Geometry: final body of the model. Coordinates: model frame, mm. A direction names the side the tool comes from. Give positions to 0.01 mm unless a question says otherwise; leave off trailing zeros. Loops run counter-clockwise (first coordinate to the right, second up) from the corner with the lowest first, then second, coordinate; pieces in that order, holes last. Notation, with made-up numbers: (4, -38) -> (29, -38) arc R18 ccw to (29, -7) -> close; hole circle Ø7 at (-30.5, 24.25). An arc over 180 degrees is marked (long way). One line per item, written item: value. Start each with the question number.
from build123d import *
from build123d.topology import SkipClean

# Parameters (mm, degrees)
SALIENTE_EXTRUIR1_DEPTH    = 2.4
CORTAR_EXTRUIR1_DEPTH      = 43.673293756
CORTAR_EXTRUIR1_DEPTH_BACK = 43.673293756
CROQUIS2_R                 = 1.5
CROQUIS3_R                 = 1.5
SALIENTE_EXTRUIR2_DEPTH    = 7.5
CORTAR_EXTRUIR2_DEPTH      = 3.1
REDONDEO1_R                = 2


with BuildPart() as part:
    # Croquis1 → Saliente-Extruir1 (new, symmetric)
    with BuildSketch(Plane(origin=(0, 0, 0), x_dir=(0, 0, -1), z_dir=(1, 0, 0))):
        with BuildLine():
            Line((-41.5, 3), (41.5, 3))
            ThreePointArc((41.5, 3), (42.207106781, 2.707106781), (42.5, 2))
            Line((42.5, 2), (42.5, -2))
            ThreePointArc((42.5, -2), (42.207106781, -2.707106781), (41.5, -3))
            Line((41.5, -3), (-41.5, -3))
            ThreePointArc((-41.5, -3), (-42.207106781, -2.707106781), (-42.5, -2))
            Line((-42.5, -2), (-42.5, 2))
            ThreePointArc((-42.5, 2), (-42.207106781, 2.707106781), (-41.5, 3))
        make_face()
    extrude(amount=SALIENTE_EXTRUIR1_DEPTH, both=True)

    # Croquis2 → Cortar-Extruir1 (cut, two sides: drawn at the far end of the back side and taken through both)
    with BuildSketch(Plane(origin=(0, 0, 0), x_dir=(0, 0, -1), z_dir=(1, 0, 0)).offset(-CORTAR_EXTRUIR1_DEPTH_BACK)):
        with Locations((-39.5, 0)):
            Circle(CROQUIS2_R)
        with Locations((33.5, 0)):
            Circle(CROQUIS2_R)
    extrude(amount=CORTAR_EXTRUIR1_DEPTH + CORTAR_EXTRUIR1_DEPTH_BACK, mode=Mode.SUBTRACT)

    # Croquis3 → Saliente-Extruir2 (add, symmetric)
    with SkipClean():  # the faces are left unmerged after this step: merging them gives an invalid solid
        with BuildSketch(Plane(origin=(0, 0, 0), x_dir=(0, 0, -1), z_dir=(1, 0, 0))):
            with BuildLine():
                Line((-42.5, 2), (-42.5, -2))
                ThreePointArc((-42.5, -2), (-42.207106781, -2.707106781), (-41.5, -3))
                Line((-41.5, -3), (-27.5, -3))
                Line((-27.5, -3), (-27.5, 3))
                Line((-27.5, 3), (-41.5, 3))
                ThreePointArc((-41.5, 3), (-42.207106781, 2.707106781), (-42.5, 2))
            make_face()
            with Locations((-39.5, 0)):
                Circle(CROQUIS3_R, mode=Mode.SUBTRACT)
        extrude(amount=SALIENTE_EXTRUIR2_DEPTH, both=True)
    add(part.part.scale(1), mode=Mode.REPLACE)  # the faces are merged on a copy

    # Croquis4 → Cortar-Extruir2 (cut, symmetric)
    with BuildSketch(Plane(origin=(0, 0, 0), x_dir=(0, 0, -1), z_dir=(1, 0, 0))):
        with BuildLine():
            Line((-41.5, 3), (-34.5, 3))
            Line((-34.5, 3), (-34.5, -3))
            Line((-34.5, -3), (-41.5, -3))
            ThreePointArc((-41.5, -3), (-42.207106781, -2.707106781), (-42.5, -2))
            Line((-42.5, -2), (-42.5, 2))
            ThreePointArc((-42.5, 2), (-42.207106781, 2.707106781), (-41.5, 3))
        make_face()
    extrude(amount=CORTAR_EXTRUIR2_DEPTH, both=True, mode=Mode.SUBTRACT)

    # Redondeo1
    redondeo1_edges = [part.edges().sort_by_distance(p)[0] for p in [
        (-2.4, 0, 27.5),
        (2.4, 0, 27.5),
        (-7.5, 0, 27.5),
        (7.5, 0, 27.5),
    ]]
    fillet(redondeo1_edges, radius=REDONDEO1_R)


solid = part.part
Item 1: Mould query, pull axis Z, two halves, no side actions, for faces 4 (the face through (0, -0.9, -32.3)), 5 (the face through (6.9, 0.04, 28.07)), 6 (the face through (-2.4, 0, -9)). Classes: pulls with the +Z half, pulls with the -Z half, needs draft (parallel to the pull), parting line crosses it, or undercut.
Item 2: Access query for faces 1 (the face through (7.5, 0, 36)), 2 (the face through (2.4, 0, -9)), 3 (the face through (0, 0, 34.5)). Directions: +Z, -Z, +X, -X, +Y, -Y. A direction counts if a zero-diameter tool reaches every point of the face in a straight line with its end or side. Return the directions, or none.
Item 3: Pin query (flat end, axial travel): pin 1 (3 mm diameter, centred on y = -0.5, z = 4, fed in from -X); pin 2 (0.6 mm diameter, centred on x = -5, y = -1, fed in from -Z); pin 3 (2 mm diameter, centred on x = 0, y = 2, fed in from +Z); pin 4 (1.8 mm diameter, centred on y = 0, z = 39.5, fed in from -X). Return the tip coordinate at first contact, or that it passes through.
Item 4: Section D-D, the plane z = -3.5. Output: boundary loops of the cut face in (x, y), then the cut area to 3 significant figures.
Item 5: Ray query, line 1 along Y through (x, z) = (-5.5, 39.5); line 2 along Z through (x, y) = (0.4, 0); line 3 along X through (y, z) = (2.75, 0.5). Return the intervals inside material, ascending. Write a range as [from, to].
Item 6: Section C-C, the plane x = 1.25. Output: boundary loops of the cut face in (y, z).
Item 7: Section A-A, the plane z = 39.5. Output: boundary loops of the cut face in (x, y), then the cut area to 3 significant figures.
Item 8: Section B-B, the plane y = 0. Output: boundary loops of the cut face in (x, z).
Geometry check:
1. face 4: undercut
1. face 5: pulls with the -Z half
1. face 6: needs draft
2. face 1: +Z, -Z, +X, +Y, -Y
2. face 2: -Z, +X, +Y, -Y
2. face 3: +Z, +Y, -Y
3. pin 1: stops at x = -2.4
3. pin 2: stops at z = 27.5
3. pin 3: stops at z = 34.5
3. pin 4: passes through
4. outline: (-2.4, -3) -> (2.4, -3) -> (2.4, 3) -> (-2.4, 3) -> close
4. area: 28.8 mm2
5. line 1: y = [-3, -1.5], [1.5, 3]
5. line 2: z = [-42.5, -35], [-32, 34.5]
5. line 3: x = [-2.4, 2.4]
6. outline: (-3, -41.5) arc R1 ccw to (-2, -42.5) -> (2, -42.5) arc R1 ccw to (3, -41.5) -> (3, 34.5) -> (-3, 34.5) -> close; hole circle Ø3 at (0, -33.5)
7. outline: (-7.5, -3) -> (-3.1, -3) -> (-3.1, -1.5) -> (-7.5, -1.5) -> close; (-7.5, 1.5) -> (-3.1, 1.5) -> (-3.1, 3) -> (-7.5, 3) -> close; (3.1, -3) -> (7.5, -3) -> (7.5, -1.5) -> (3.1, -1.5) -> close; (3.1, 1.5) -> (7.5, 1.5) -> (7.5, 3) -> (3.1, 3) -> close
7. area: 26.4 mm2
8. outline: (-7.5, 29.5) arc R2 ccw to (-5.5, 27.5) -> (-4.4, 27.5) arc R2 cw to (-2.4, 25.5) -> (-2.4, -32) -> (2.4, -32) -> (2.4, 25.5) arc R2 cw to (4.4, 27.5) -> (5.5, 27.5) arc R2 ccw to (7.5, 29.5) -> (7.5, 38) -> (3.1, 38) -> (3.1, 34.5) -> (-3.1, 34.5) -> (-3.1, 38) -> (-7.5, 38) -> close; (-7.5, 41) -> (-3.1, 41) -> (-3.1, 42.5) -> (-7.5, 42.5) -> close; (-2.4, -42.5) -> (2.4, -42.5) -> (2.4, -35) -> (-2.4, -35) -> close; (3.1, 41) -> (7.5, 41) -> (7.5, 42.5) -> (3.1, 42.5) -> close
